The model under review builds one solid part; all positions refer to its coordinate system, in mm. Face numbers are marked on the shaded views. A direction names the side the tool comes from. Round coordinates to 2 decimals unless told otherwise and drop trailing zeros. Loops run counter-clockwise (first coordinate to the right, second up) from the corner with the lowest first, then second, coordinate; pieces in that order, holes last. Notation, with made-up numbers: M 83.5,40 L 116.5,40 A31 ccw 116.5,72 Z; hole C -26,-20.75 d4. An arc over 180 degrees is marked long. One line per question, with ' | ' between items.
from build123d import *

# Parameters (mm, degrees)
SKETCH1_W           = 30
SKETCH1_H           = 2.5
SKETCH3_R           = 2.5
BOSS_EXTRUDE2_DEPTH = 2.5


with BuildPart() as part:
    # Sketch1 → Revolve-Thin1 (revolve)
    with BuildSketch(Plane.XY):
        with Locations((0, 1.25)):
            Rectangle(SKETCH1_W, SKETCH1_H)
    revolve(axis=Axis((-15, 0, 0), (1, 0, 0)))

    # Sketch3 → Boss-Extrude2 (add)
    with BuildSketch(Plane.XY):
        with BuildLine():
            Line((15, 2.5), (15, -2.5))
            ThreePointArc((15, -2.5), (28.538348415, 0), (15, 2.5))
        make_face()
        with Locations((21.538348415, 0)):
            Circle(SKETCH3_R, mode=Mode.SUBTRACT)
        with BuildLine():
            Line((-15, -2.5), (-15, 2.5))
            ThreePointArc((-15, 2.5), (-28.538348415, 0), (-15, -2.5))
        make_face()
        with Locations((-21.538348415, 0)):
            Circle(SKETCH3_R, mode=Mode.SUBTRACT)
    extrude(amount=-BOSS_EXTRUDE2_DEPTH)


solid = part.part
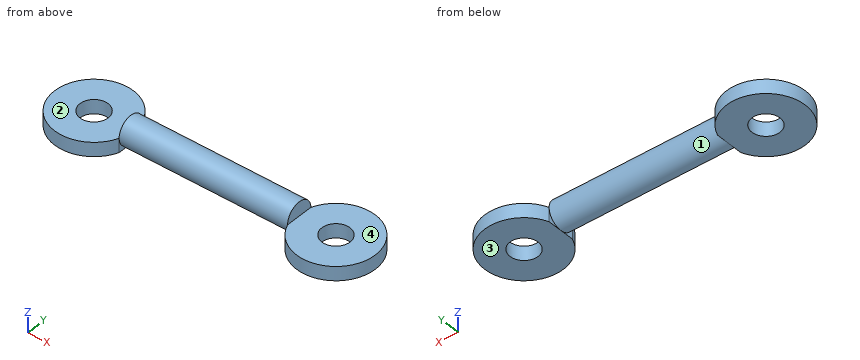
1) Mouldability with a two-part tool opening along X and no side actions: class the marked faces 1 and 2 as +X half, -X half, draft (parallel to the pull), parting line (faces both ways), or undercut.
Output values:
face 1: undercut | face 2: draft
2) Add section D-D on x = -9. State the section outline as (y, z) points, then the cut area to 3 significant figures.
Output values:
outline: C 0,0 d5 | area: 19.6 mm²
3) Insertion check: P1, Ø6.5, axis at x = 21.54, y = 0, coming from the -Z side; P2, Ø1, axis at y = -4, z = 2, coming from the +X side; P3, Ø1.2, axis at y = 1, z = -2, coming from the -X side; P4, Ø0.8, axis at y = 1.5, z = -1.5, coming from the +X side. Each pin has a flat end and moves straight along its axis. Give the tip position at first contact, or say it passes through.
Output values:
P1: stops at z = -2.5 | P2: passes through | P3: stops at x = -28.53 | P4: stops at x = 28.45
4) Add section B-B on z = -1.2. State the section outline as (x, y) points, then the cut area to 3 significant figures.
Output values:
outline: M -15,-2.5 L -15,-2.19 L 15,-2.19 L 15,-2.5 A7 ccw long 15,2.5 L 15,2.19 L -15,2.19 L -15,2.5 A7 ccw long Z; hole C -21.54,0 d5; hole C 21.54,0 d5 | area: 397 mm²
5) Machinability: for the marked faces 3 and 4, which of the approach directions +Z, -Z, +X, -X, +Y, -Y give a long, thin tool a straight path to every point of the face, cutting with its end or side? Answer none if there is none.
Output values:
face 3: -Z, +X, -X, +Y, -Y | face 4: +Z, +X, +Y, -Y
6) Add section A-A on y = 5. State the section outline as (x, z) points.
Output values:
outline: M -26.44,-2.5 L -16.64,-2.5 L -16.64,0 L -26.44,0 Z; M 16.64,-2.5 L 26.44,-2.5 L 26.44,0 L 16.64,0 Z
7) Add section C-C on y = 1.5. State the section outline as (x, z) points, then the cut area to 3 significant figures.
Output values:
outline: M -28.38,-2.5 L -23.54,-2.5 L -23.54,0 L -28.38,0 Z; M -19.54,-2.5 L -15,-2.5 L -15,-2 L 15,-2 L 15,-2.5 L 19.54,-2.5 L 19.54,0 L 15,0 L 15,2 L -15,2 L -15,0 L -19.54,0 Z; M 23.54,-2.5 L 28.38,-2.5 L 28.38,0 L 23.54,0 Z | area: 167 mm²
8) For line 1 (X direction, y = 0.25, z = -2.05); line 2 (X direction, y = 1.25, z = -2.05); line 3 (X direction, y = 5.25, z = -1.45), list the stretches that pass through material, from the lowest coordinate up.
Output values:
line 1: x = -28.53 to -24.03, -19.05 to 19.05, 24.03 to 28.53 | line 2: x = -28.43 to -23.7, -19.37 to 19.37, 23.7 to 28.43 | line 3: x = -26.17 to -16.91, 16.91 to 26.17
